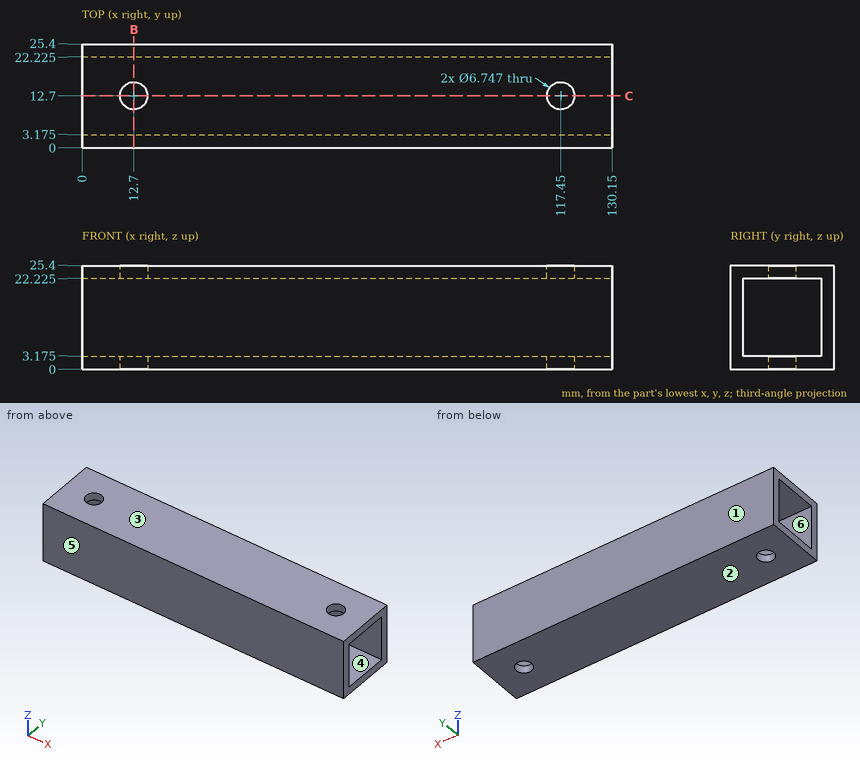
Design review of the part shown in the three views and the two pictorial views. Dimensions are in mm from the part's minimum x, y and z. A direction names the side the tool comes from. Round coordinates to 2 decimals unless told otherwise and drop trailing zeros. Write each loop counter-clockwise with the first axis right and the second up, starting at its lowest first coordinate (ties: lowest second). Pieces come first, ordered by that corner, then holes. Notation, with made-up numbers: (80.5, -35.75) - (100.5, -35.75) arc R23 cw to (100.5, -26.75) - close; hole circle Ø5 at (-3, 89.5). An arc over 180 degrees is marked (long way). Return JSON: item names as keys, results as strings. Group by question number.
Item 1: We need section C-C on y = 12.7. Give the number of separate pieces and of enclosed holes in the cut face.
Item 2: Machinability: for the marked faces 5 and 6, which of the approach directions +Z, -Z, +X, -X, +Y, -Y give a long, thin tool a straight path to every point of the face, cutting with its end or side? Answer none if there is none.
Item 3: We need section B-B on x = 12.7. Write out the cut boundary in (y, z) (1 decimal).
Item 4: The part is to be moulded in two halves that separate along Z. For the marked faces 1, 2, 3 and 4, say which applies: pulls with the +Z half, pulls with the -Z half, needs draft (parallel to the pull), parting line crosses it, or undercut.
Item 5: For probe 1 along Y at (x, z) = (75.5, 4.25) (1 decimal); probe 2 along Y at (x, z) = (12.7, 23.35), list the stretches that pass through material, from the lowest coordinate up. Write a range as [from, to].
Model answer:
{
 "1": {"separate pieces": "6", "enclosed holes": "0"},
 "2": {"face 5": "+Z, -Z, +X, -X, -Y", "face 6": "+X, -X"},
 "3": {"outline": "(0, 0) - (9.3, 0) - (9.3, 3.2) - (3.2, 3.2) - (3.2, 22.2) - (9.3, 22.2) - (9.3, 25.4) - (0, 25.4) - close; (16.1, 0) - (25.4, 0) - (25.4, 25.4) - (16.1, 25.4) - (16.1, 22.2) - (22.2, 22.2) - (22.2, 3.2) - (16.1, 3.2) - close"},
 "4": {"face 1": "needs draft", "face 2": "pulls with the -Z half", "face 3": "pulls with the +Z half", "face 4": "undercut"},
 "5": {"probe 1": "y = [0, 3.2], [22.2, 25.4]", "probe 2": "y = [0, 9.33], [16.07, 25.4]"}
}
